Autodesk Inventor part; units mm, degrees
ref_plane "YZ Plane" through (0, 0, 0) normal (1, 0, 0) x (0, 1, 0)
ref_plane "XZ Plane" through (0, 0, 0) normal (0, 1, 0) x (-1, 0, 0)
ref_plane "XY Plane" through (0, 0, 0) normal (0, 0, 1) x (1, 0, 0)
sketch "Sketch1" plane through (0, 0, 0) normal (0, 1, 0) x (-1, 0, 0)
  circle A0 centre (0, 0) radius 46
  circle A1 centre (0, 0) radius 49
  dimension "d0" = 92
  dimension "d1" = 98
extrude "Extrusion1" add sketch "Sketch1" along normal blind 50
chamfer "Chamfer1" distance 2 angle 45 1 edges at (49, 50, 0)
chamfer "Chamfer2" distance 1 angle 45 1 edges at (46, 0, 0)
sketch "Sketch2" plane through (0, 0, 0) normal (1, 0, 0) x (0, 1, 0)
  circle A0 centre (30, 0) radius 2.5
  line L0 (50, 46) -> (50, -46)
  point P0 (0, 0)
  dimension "d10" = 5
  dimension "d11" = 20
extrude "Extrusion2" cut sketch "Sketch2" along normal through all both and the other way through all
properties part number "HubSparHole90"
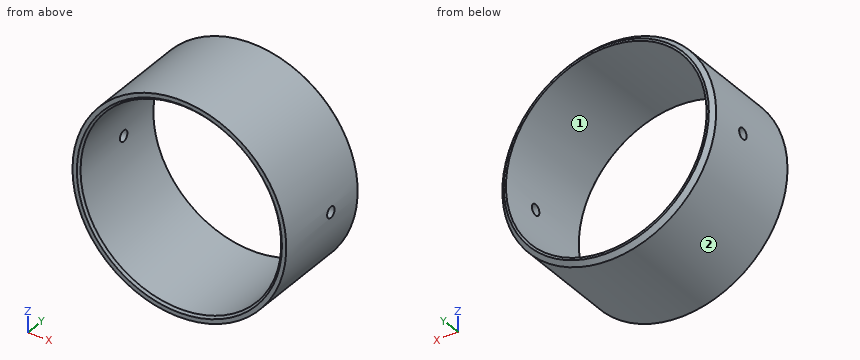
CAD build for the part. Positions are in the model's coordinates, mm. Face numbers are marked on the shaded views. Give positions to 0.01 mm unless a question says otherwise; leave off trailing zeros. Loops run counter-clockwise (first coordinate to the right, second up) from the corner with the lowest first, then second, coordinate; pieces in that order, holes last. Notation, with made-up numbers: (14, 42) - (60, 42) arc R11 ccw to (60, 63) - close; hole circle Ø7 at (-20, 34.25). An arc over 180 degrees is marked (long way). Put each result on its own line as item: value.
Q1. Slice it at B-B (z = 0). Give the cut face in (x, y).
Filled in:
outline: (-49, 0) - (-47, 0) - (-46, 1) - (-46, 27.5) - (-49, 27.5) - close; (-49, 32.5) - (-46, 32.5) - (-46, 50) - (-47, 50) - (-49, 48) - close; (46, 1) - (47, 0) - (49, 0) - (49, 27.5) - (46, 27.5) - close; (46, 32.5) - (49, 32.5) - (49, 48) - (47, 50) - (46, 50) - close
Q2. Flat gauge pins, fed straight in: pin 1 (6 mm diameter, centred on y = 20.5, z = -7, fed in from -X); pin 2 (2 mm diameter, centred on x = -7.5, y = 23.5, fed in from +Z); pin 3 (3 mm diameter, centred on x = -11.5, y = 41.5, fed in from +Z). Where does each tip first touch, or does it go through?
Filled in:
pin 1: stops at x = -48.84
pin 2: stops at z = 48.57
pin 3: stops at z = 47.97
Q3. Slice it at D-D (y = 17.5). Give the cut face in (x, z).
Filled in:
outline: circle Ø98 at (0, 0); hole circle Ø92 at (0, 0)
Q4. Probe line 1 along X through (y, z) = (24.5, 0); line 2 along Z through (x, y) = (16.5, 38); line 3 along X through (y, z) = (47.5, -39). List the from-to ranges inside material, lowest first.
Filled in:
line 1: x = -49 to -46, 46 to 49
line 2: z = -46.14 to -42.94, 42.94 to 46.14
line 3: x = -29.66 to -24.39, 24.39 to 29.66
Q5. Slice it at A-A (x = 0). Give the cut face in (y, z), plus the area to 3 significant figures.
Filled in:
outline: (0, -49) - (48, -49) - (50, -47) - (50, -46) - (1, -46) - (0, -47) - close; (0, 47) - (1, 46) - (50, 46) - (50, 47) - (48, 49) - (0, 49) - close
area: 295 mm²
Q6. Mould opens along X. For the marked faces 1 and 2 say: pulls with the +X half, pulls with the -X half, needs draft (parallel to the pull), parting line crosses it, or undercut.
Filled in:
face 1: undercut
face 2: parting line crosses it
